Can you work these out from the model? Positions are in its coordinate system, mm. A direction names the side the tool comes from. Coordinates: 2 decimals unless noted, no trailing zeros. Order: outer loops, then holes, each group sorted by start corner. A loop starts at its lowest first (then second) coordinate and runs counter-clockwise, first axis right, second up. Notation, with made-up numbers: (-17.75, -2.5) -> (9.25, -2.5) arc R20 ccw to (9.25, 9.5) -> close; hole circle Ø7 at (3.25, 60). An arc over 180 degrees is marked (long way). Answer in a Markdown table with one row per item. Add a question column.
1. We'd pull the mould along Z, two halves only. Please class faces 1 (the face through (-19, 8, -12)), 2 (the face through (7, 17.3, -10)), 3 (the face through (-28.6, 9.86, 11.55)): pulls with the +Z half, pulls with the -Z half, needs draft (parallel to the pull), parting line crosses it, or undercut.
2. Imagine slicing it at A-A on z = -10. State how many separate pieces and enclosed holes the cut face has, plus the area to 3 significant figures.
3. Will these pins go through, and if not, where does the flat tip stop? pin 1 (5 mm diameter, centred on x = -4, z = 2, fed in from +Y); pin 2 (1.6 mm diameter, centred on x = 8.5, z = -9, fed in from +Y).
4. If I drill on line 1 along Z through (x, y) = (-29.15, 17.5); line 2 along Z through (x, y) = (-24.15, 17.8); line 3 along X through (y, z) = (18, -3.5), over which ranges is the centre line in solid material (lowest first)? Write a range as [from, to].
5. Imagine slicing it at B-B on x = -17. Write out the boundary of the cut face in (y, z).
6. On a 3-axis mill with a long thin cutter (end or side, diameter ignored), from which of +Z, -Z, +X, -X, +Y, -Y can I reach the whole of each face in a straight line? I mean faces 4 (the face through (28.7, 9.86, 11.45)), 5 (the face through (10.58, 18.67, -12.37)), 6 (the face through (19.507, 9, -10)). Say none if no direction works.
7. Imagine slicing it at D-D on z = 2.95. Write out the boundary of the cut face in (x, y).
from build123d import *

# Parameters (mm, degrees)
SKETCH1_W             = 64.3
SKETCH1_H             = 30
BOSS_EXTRUDE1_DEPTH   = 20
VARILLAS_START        = 20
SKETCH1_3_R           = 8.05
SKETCH1_3_R_2         = 8.1
SKETCH1_3_R_3         = 8
VARILLAS_HUECAS_DEPTH = 15
TORNILLOS_START       = 20
SKETCH1_4_R           = 1.35
SKETCH1_4_R_2         = 1.4
SKETCH1_4_R_3         = 1.3
TORNILLOS_ALEM_DEPTH  = 12
TORNILLOS_PCB_DEPTH   = 2.7
SKETCH1_5_R           = 2
SKETCH1_5_R_2         = 2.05
SKETCH1_5_R_3         = 2.1
VARILLAS_SERVOS_DEPTH = 20
CHAMFER1_SIZE         = 7
CUT_EXTRUDE5_REACH    = 41.47
CUT_EXTRUDE6_START    = 20
SKETCH1_7_R           = 1.35
SKETCH1_7_R_2         = 1.3
SKETCH1_7_R_3         = 1.4
CUT_EXTRUDE6_DEPTH    = 3.5


with BuildPart() as part:
    # Sketch1 → Boss-Extrude1 (new body)
    with BuildSketch(Plane(origin=(0, 0, 0), x_dir=(1, 0, 0), z_dir=(0, 1, 0))):
        Rectangle(SKETCH1_W, SKETCH1_H)
    extrude(amount=BOSS_EXTRUDE1_DEPTH)

    # Sketch1<3> → Varillas huecas (cut)
    with BuildSketch(Plane(origin=(0, 0, 0), x_dir=(1, 0, 0), z_dir=(0, 1, 0)).offset(VARILLAS_START)):
        with Locations(Location((-0.1, -2.95, 0), (0, 0, 90))):
            Circle(SKETCH1_3_R)
        with Locations(Location((20.05, -2.95, 0), (0, 0, 90))):
            Circle(SKETCH1_3_R_2)
        with Locations(Location((-20.15, -2.95, 0), (0, 0, 90))):
            Circle(SKETCH1_3_R_3)
    extrude(amount=-VARILLAS_HUECAS_DEPTH, mode=Mode.SUBTRACT)

    # Sketch1<4> → Tornillos Alem (cut)
    with BuildSketch(Plane(origin=(0, 0, 0), x_dir=(1, 0, 0), z_dir=(0, 1, 0)).offset(TORNILLOS_START)):
        with Locations(Location((-24.15, 12, 0), (0, 0, 90))):
            Circle(SKETCH1_4_R)
        with Locations(Location((-19.15, 12, 0), (0, 0, 90))):
            Circle(SKETCH1_4_R_2)
        with Locations(Location((-29.15, 12, 0), (0, 0, 90))):
            Circle(SKETCH1_4_R_3)
    extrude(amount=-TORNILLOS_ALEM_DEPTH, mode=Mode.SUBTRACT)

    # Sketch1<6> → Tornillos PCB (cut)
    with BuildSketch(Plane(origin=(0, 0, 0), x_dir=(1, 0, 0), z_dir=(0, 1, 0)).offset(TORNILLOS_START)):
        Polygon((9.185714286, 6.824573519), (11.935714286, 8.41228676), (11.935714286, 11.58771324), (9.185714286, 13.175426481), (6.435714286, 11.58771324), (6.435714286, 8.41228676), align=None)
        Polygon((17.707142857, 6.766838493), (20.507142857, 8.383419246), (20.507142857, 11.616580754), (17.707142857, 13.233161507), (14.907142857, 11.616580754), (14.907142857, 8.383419246), align=None)
        Polygon((26.328571429, 6.709103466), (29.178571429, 8.354551733), (29.178571429, 11.645448267), (26.328571429, 13.290896534), (23.478571429, 11.645448267), (23.478571429, 8.354551733), align=None)
    extrude(amount=-TORNILLOS_PCB_DEPTH, mode=Mode.SUBTRACT)

    # Sketch1<5> → Varillas servos (cut)
    with BuildSketch(Plane(origin=(0, 0, 0), x_dir=(1, 0, 0), z_dir=(0, 1, 0)).offset(VARILLAS_START)):
        with Locations(Location((-12.778571429, 10, 0), (0, 0, 90))):
            Circle(SKETCH1_5_R)
        with Locations(Location((-5.757142857, 10, 0), (0, 0, 90))):
            Circle(SKETCH1_5_R_2)
        with Locations(Location((1.364285714, 10, 0), (0, 0, 90))):
            Circle(SKETCH1_5_R_3)
    extrude(amount=-VARILLAS_SERVOS_DEPTH, mode=Mode.SUBTRACT)

    # Chamfer1
    chamfer1_edges = [part.edges().sort_by_distance(p)[0] for p in [
        (-32.15, 10, 15),
        (32.15, 10, 15),
    ]]
    chamfer(chamfer1_edges, length=CHAMFER1_SIZE)

    # Sketch2 → Cut-Extrude5 (cut, up to next)
    with BuildSketch(Plane(origin=(0, 17.3, 0), x_dir=(1, 0, 0), z_dir=(0, 1, 0)), mode=Mode.PRIVATE) as cut_extrude5_sk1:
        Polygon((24.478571429, 11.068097998), (24.478571429, 8.931902002), (26.328571429, 7.863804004), (28.178571429, 8.931902002), (28.178571429, 11.068097998), (26.328571429, 12.136195996), align=None)
    cut_extrude5_tool1 = extrude(cut_extrude5_sk1.sketch, amount=-CUT_EXTRUDE5_REACH, mode=Mode.PRIVATE) & part.part
    # Sketch2 → Cut-Extrude5 (cut, up to next)
    with BuildSketch(Plane(origin=(0, 17.3, 0), x_dir=(1, 0, 0), z_dir=(0, 1, 0)), mode=Mode.PRIVATE) as cut_extrude5_sk2:
        Polygon((15.907142857, 11.039230485), (15.907142857, 8.960769515), (17.707142857, 7.921539031), (19.507142857, 8.960769515), (19.507142857, 11.039230485), (17.707142857, 12.078460969), align=None)
    cut_extrude5_tool2 = extrude(cut_extrude5_sk2.sketch, amount=-CUT_EXTRUDE5_REACH, mode=Mode.PRIVATE) & part.part
    # Sketch2 → Cut-Extrude5 (cut, up to next)
    with BuildSketch(Plane(origin=(0, 17.3, 0), x_dir=(1, 0, 0), z_dir=(0, 1, 0)), mode=Mode.PRIVATE) as cut_extrude5_sk3:
        Polygon((10.935714286, 11.010362971), (9.185714286, 12.020725942), (7.435714286, 11.010362971), (7.435714286, 8.989637029), (9.185714286, 7.979274058), (10.935714286, 8.989637029), align=None)
    cut_extrude5_tool3 = extrude(cut_extrude5_sk3.sketch, amount=-CUT_EXTRUDE5_REACH, mode=Mode.PRIVATE) & part.part
    add(cut_extrude5_tool1.solids().sort_by_distance((26.328571, 17.3, -10))[0], mode=Mode.SUBTRACT)
    add(cut_extrude5_tool2.solids().sort_by_distance((17.707143, 17.3, -10))[0], mode=Mode.SUBTRACT)
    add(cut_extrude5_tool3.solids().sort_by_distance((9.185714, 17.3, -10))[0], mode=Mode.SUBTRACT)

    # Sketch1<7> → Cut-Extrude6 (cut)
    with BuildSketch(Plane(origin=(0, 0, 0), x_dir=(1, 0, 0), z_dir=(0, 1, 0)).offset(CUT_EXTRUDE6_START)):
        with Locations(Location((-24.15, 8, 0), (0, 0, 90))):
            Circle(SKETCH1_7_R)
        with Locations(Location((-29.15, 8, 0), (0, 0, 90))):
            Circle(SKETCH1_7_R_2)
        with Locations(Location((-19.15, 8, 0), (0, 0, 90))):
            Circle(SKETCH1_7_R_3)
    extrude(amount=-CUT_EXTRUDE6_DEPTH, mode=Mode.SUBTRACT)


solid = part.part
Answers follow:
| question | item | result |
|---|---|---|
| 1 | face 1 | undercut |
| 1 | face 2 | undercut |
| 1 | face 3 | pulls with the +Z half |
| 2 | separate pieces | 7 |
| 2 | enclosed holes | 0 |
| 2 | area | 808 mm² |
| 3 | pin 1 | stops at y = 5 |
| 3 | pin 2 | stops at y = 17.3 |
| 4 | line 1 | z = [-15, -13.3], [-10.7, -9.3], [-6.7, 11] |
| 4 | line 2 | z = [-15, -13.35], [-10.65, -9.35], [-6.65, -3.98], [9.88, 15] |
| 4 | line 3 | x = [-32.15, -24.88], [-15.42, -4.92], [4.72, 15.15], [24.95, 32.15] |
| 5 | outline | (0, -15) -> (20, -15) -> (20, -4.4) -> (5, -4.4) -> (5, 10.3) -> (20, 10.3) -> (20, 15) -> (0, 15) -> close |
| 6 | face 4 | +Z, +X, +Y, -Y |
| 6 | face 5 | +Y |
| 6 | face 6 | +Y, -Y |
| 7 | outline | (-32.15, 0) -> (32.15, 0) -> (32.15, 20) -> (28.15, 20) -> (28.15, 5) -> (11.95, 5) -> (11.95, 20) -> (7.95, 20) -> (7.95, 5) -> (-8.15, 5) -> (-8.15, 20) -> (-12.15, 20) -> (-12.15, 5) -> (-28.15, 5) -> (-28.15, 20) -> (-32.15, 20) -> close |
